Source: CAD feature listing. Evaluate the final solid. Frame: model axes, mm. A direction names the side the tool comes from. Give positions to 0.01 mm unless a question says otherwise; leave off trailing zeros. Order: outer loops, then holes, each group sorted by start corner. A loop starts at its lowest first (then second) coordinate and runs counter-clockwise, first axis right, second up. Notation, with made-up numbers: (23.5, 79.25) - (71.5, 79.25) arc R30 ccw to (71.5, 102.25) - close; hole circle Ø7 at (-19, 36.5). An arc over 180 degrees is marked (long way). Write each question's results on one line, items separated by ' | '. Start each with the question number.
Item 1: Set-up query: faces 1 (the flat face through (-32, 4, 5.6)), 2 (the flat face through (36.2, -1.4, 5)), 3 (the cylindrical face through (26.755, 0.209, 5.069)), 4 (the cylindrical face through (34.247, 0.121, 0.986)). Return all of +Z, -Z, +X, -X, +Y, -Y with unobstructed straight access to the full face (end or side cutting, diameter ignored); none if empty.
Item 2: Contact query for flat-ended pins moving along their axis: pin 1 Ø2.5 at (x, y) = (-33.5, -1.5) entering from +Z; pin 2 Ø8 at (y, z) = (1.5, 44) entering from -X; pin 3 Ø4 at (x, y) = (34.5, -2) entering from +Z. Output: stop coordinate, or through.
Item 3: Section B-B on y = 1.25. State how many separate pieces and enclosed holes the cut face has, and give its area (3 significant figures).
Item 4: Line query: line 1 along X through (y, z) = (0, 34.5); line 2 along X through (y, z) = (-1.5, 20.5); line 3 along X through (y, z) = (0.25, 4). Output: solid intervals per line, ascending.
Item 5: Mould query, pull axis X, two halves, no side actions, for faces 5 (the flat face through (-26.5, 0, 32)), 6 (the cylindrical face through (26.813, -2.082, 12.518)), 7 (the flat face through (31, 4.75, 6)), 8 (the cylindrical face through (18.354, 0.676, 27.185)). Classes: released by +X, released by -X, zero draft, split by the parting line, or undercut.
Item 6: Section A-A on y = -6. Output: boundary loops of the cut face in (x, z).
```python
from build123d import *

# Parameters (mm, degrees)
SKETCH_1_W                     = 53
SKETCH_1_H                     = 20
EXTRUDE_1_DEPTH                = 50
HOLE_WIZARD_M5_1_D             = 4.5
HOLE_WIZARD_M5_1_DEPTH         = 45
HOLE_WIZARD_M5_1_TIP           = 1.351936393
SKETCH_4_W                     = 5
SKETCH_4_H                     = 20
EXTRUDE_2_DEPTH                = 20
HOLE_WIZARD_M4_1_D             = 4.5
HOLE_WIZARD_M4_1_DEPTH         = 15
HOLE_WIZARD_M4_1_CBORE_D       = 8
HOLE_WIZARD_M4_1_CBORE_DEPTH   = 3
HOLE_WIZARD_M4_1_TIP           = 1.351936393
SKETCH_7_W                     = 5
SKETCH_7_H                     = 20
EXTRUDE_3_DEPTH                = 20
HOLE_WIZARD_M5_1_2_D           = 5.5
HOLE_WIZARD_M5_1_2_DEPTH       = 15
HOLE_WIZARD_M5_1_2_CBORE_D     = 9.5
HOLE_WIZARD_M5_1_2_CBORE_DEPTH = 3
HOLE_WIZARD_M5_1_2_TIP         = 1.652366702
FILLET_1_R                     = 10
SKETCH_10_W                    = 6
SKETCH_10_H                    = 8
SKETCH_10_W_2                  = 7
SKETCH_10_H_2                  = 9.5
CUT_EXTRUDE_1_DEPTH            = 20
SKETCH_11_W                    = 10
SKETCH_11_H                    = 20
CUT_EXTRUDE_2_DEPTH            = 10


with BuildPart() as part:
    # 스케치1 → 보스-돌출1 (new body)
    with BuildSketch(Plane.XY):
        Rectangle(SKETCH_1_W, SKETCH_1_H)
    extrude(amount=EXTRUDE_1_DEPTH)

    # Hole Wizard M5 _ _1
    with Locations(Plane.XY.offset(50)):
        with Locations((20.5, 0), (-20.5, 0)):
            Hole(HOLE_WIZARD_M5_1_D / 2, depth=HOLE_WIZARD_M5_1_DEPTH)
            with Locations((0, 0, -(HOLE_WIZARD_M5_1_DEPTH + HOLE_WIZARD_M5_1_TIP / 2))):  # 118° drill point
                Cone(0, HOLE_WIZARD_M5_1_D / 2, HOLE_WIZARD_M5_1_TIP, mode=Mode.SUBTRACT)

    # 스케치4 → 보스-돌출2 (add)
    with BuildSketch(Plane.ZY.offset(26.5)):
        with Locations((2.5, 0)):
            Rectangle(SKETCH_4_W, SKETCH_4_H)
    extrude(amount=EXTRUDE_2_DEPTH)

    # M4 소켓 머리 캡 나사용 카운터보어1
    with Locations(Plane.XY.offset(5)):
        with Locations((-31.5, 0)):
            CounterBoreHole(HOLE_WIZARD_M4_1_D / 2, HOLE_WIZARD_M4_1_CBORE_D / 2, HOLE_WIZARD_M4_1_CBORE_DEPTH, depth=HOLE_WIZARD_M4_1_DEPTH)
            with Locations((0, 0, -(HOLE_WIZARD_M4_1_DEPTH + HOLE_WIZARD_M4_1_TIP / 2))):  # 118° drill point
                Cone(0, HOLE_WIZARD_M4_1_D / 2, HOLE_WIZARD_M4_1_TIP, mode=Mode.SUBTRACT)

    # 스케치7 → 보스-돌출3 (add)
    with BuildSketch(Plane(origin=(26.5, 0, 0), x_dir=(0, 0, -1), z_dir=(1, 0, 0))):
        with Locations((-2.5, 0)):
            Rectangle(SKETCH_7_W, SKETCH_7_H)
    extrude(amount=EXTRUDE_3_DEPTH)

    # Hole Wizard M5 _ _ _ _ _1 2
    with Locations(Plane.XY.offset(5)):
        with Locations((31.5, 0)):
            CounterBoreHole(HOLE_WIZARD_M5_1_2_D / 2, HOLE_WIZARD_M5_1_2_CBORE_D / 2, HOLE_WIZARD_M5_1_2_CBORE_DEPTH, depth=HOLE_WIZARD_M5_1_2_DEPTH)
            with Locations((0, 0, -(HOLE_WIZARD_M5_1_2_DEPTH + HOLE_WIZARD_M5_1_2_TIP / 2))):  # 118° drill point
                Cone(0, HOLE_WIZARD_M5_1_2_D / 2, HOLE_WIZARD_M5_1_2_TIP, mode=Mode.SUBTRACT)

    # 필렛1
    # the kernel refuses this fillet: 10 mm, written as the material it adds along each edge
    with BuildSketch(Plane(origin=(-26.5, 10, 5), x_dir=(0, 0, 1), z_dir=(0, -1, 0))) as fillet_1_piece_1_section:
        with BuildLine():
            CenterArc((FILLET_1_R, FILLET_1_R), FILLET_1_R, 180, 90)
            Line((0, FILLET_1_R), (0, 0))
            Line((0, 0), (FILLET_1_R, 0))
        make_face()
    fillet_1_piece_1 = extrude(amount=20, mode=Mode.PRIVATE)
    fillet_1_piece_1 = fillet_1_piece_1 - Plane(origin=(-31.5, 0, 12.39249306), x_dir=(1, 0, 0), z_dir=(0, 0, 1)) * Cylinder(4, 81, mode=Mode.PRIVATE)
    add(fillet_1_piece_1)
    with BuildSketch(Plane(origin=(26.5, 10, 5), x_dir=(0, 0, 1), z_dir=(0, -1, 0))) as fillet_1_piece_2_section:
        with BuildLine():
            CenterArc((FILLET_1_R, -FILLET_1_R), FILLET_1_R, 90, 90)
            Line((0, -FILLET_1_R), (0, 0))
            Line((0, 0), (FILLET_1_R, 0))
        make_face()
    fillet_1_piece_2 = extrude(amount=20, mode=Mode.PRIVATE)
    fillet_1_piece_2 = fillet_1_piece_2 - Plane(origin=(31.5, 0, 12.393306283), x_dir=(1, 0, 0), z_dir=(0, 0, 1)) * Cylinder(4.75, 80, mode=Mode.PRIVATE)
    add(fillet_1_piece_2)

    # 스케치10 → 컷-돌출1 (cut)
    with BuildSketch(Plane.XY.offset(5)):
        with Locations((-33.5, 0)):
            Rectangle(SKETCH_10_W, SKETCH_10_H)
        with Locations((33, 0)):
            Rectangle(SKETCH_10_W_2, SKETCH_10_H_2)
    extrude(amount=CUT_EXTRUDE_1_DEPTH, mode=Mode.SUBTRACT)

    # 스케치11 → 컷-돌출2 (cut)
    with BuildSketch(Plane.XY.offset(5)):
        with Locations((-41.5, 0)):
            Rectangle(SKETCH_11_W, SKETCH_11_H)
        with Locations((41.5, 0)):
            Rectangle(SKETCH_11_W, SKETCH_11_H)
    extrude(amount=-CUT_EXTRUDE_2_DEPTH, mode=Mode.SUBTRACT)


solid = part.part
```
Evaluation:
1) face 1: +Z, -X | face 2: +Z, +X | face 3: +Z | face 4: +Z, -Z
2) pin 1: stops at z = 2 | pin 2: stops at x = -26.5 | pin 3: stops at z = 5
3) separate pieces: 3 | enclosed holes: 0 | area: 2,350 mm^2
4) line 1: x = -26.5 to -22.75, -18.25 to 18.25, 22.75 to 26.5 | line 2: x = -26.5 to -22.18, -18.82 to 18.82, 22.18 to 26.5 | line 3: x = -36.5 to -35.49, -27.51 to -21.03, -19.97 to 19.97, 21.03 to 26.76, 36.24 to 36.5
5) face 5: released by -X | face 6: released by +X | face 7: zero draft | face 8: undercut
6) outline: (-36.5, 0) - (36.5, 0) - (36.5, 5) arc R10 cw to (26.5, 15) - (26.5, 50) - (-26.5, 50) - (-26.5, 15) arc R10 cw to (-36.5, 5) - close
